Here's the drawing with two shaded views (mm, measured from the low corner). I have some questions. A direction names the side the tool comes from. Coordinates: 2 decimals unless noted, no trailing zeros. Loops run counter-clockwise (first coordinate to the right, second up) from the corner with the lowest first, then second, coordinate; pieces in that order, holes last. Notation, with made-up numbers: (70.5, -29) -> (76.5, -29) arc R26 ccw to (76.5, 8) -> close; hole circle Ø4 at (-12, 25.5). An arc over 180 degrees is marked (long way). Answer as a JSON object with one key per item and string values. Group by question number.
1) If we mould it in two halves opening along Y, with no side actions, what happens to the marked faces 3, 4 and 5? For each: +Y half, -Y half, draft (parallel to the pull), parting line (faces both ways), or undercut.
2) I'm going to push flat-ended pins straight in: pin 1 (2 mm diameter, centred on y = 11.5, z = 7.5, fed in from -X); pin 2 (5 mm diameter, centred on y = 47.5, z = 4.5, fed in from +X); pin 3 (2 mm diameter, centred on y = 7.5, z = 4.5, fed in from +X). Where does each tip first touch, or does it pass through?
3) I want a section at A-A (y = 47.5). Write out the boundary of the cut face in (x, z).
4) I want a section at C-C (x = 2.5). Write out the boundary of the cut face in (y, z), then the cut area to 3 significant figures.
5) I want a section at B-B (z = 4.25). Write out the boundary of the cut face in (x, y), then the cut area to 3 significant figures.
6) I want a section at D-D (y = 25). Write out the boundary of the cut face in (x, z).
7) Which directions (+Z, -Z, +X, -X, +Y, -Y) give clear straight access to the entire face, cutting with the end or side of a thin tool? Please do the marked faces 1 and 2.
8) I need wall thicknesses on probe 1 along Y at (x, z) = (4.2, 4.5); probe 2 along Y at (x, z) = (0.75, 4.5); probe 3 along Z at (x, y) = (3.4, 7.5). Which ranges of each line are inside material? Lowest first, please. Write a range as [from, to].
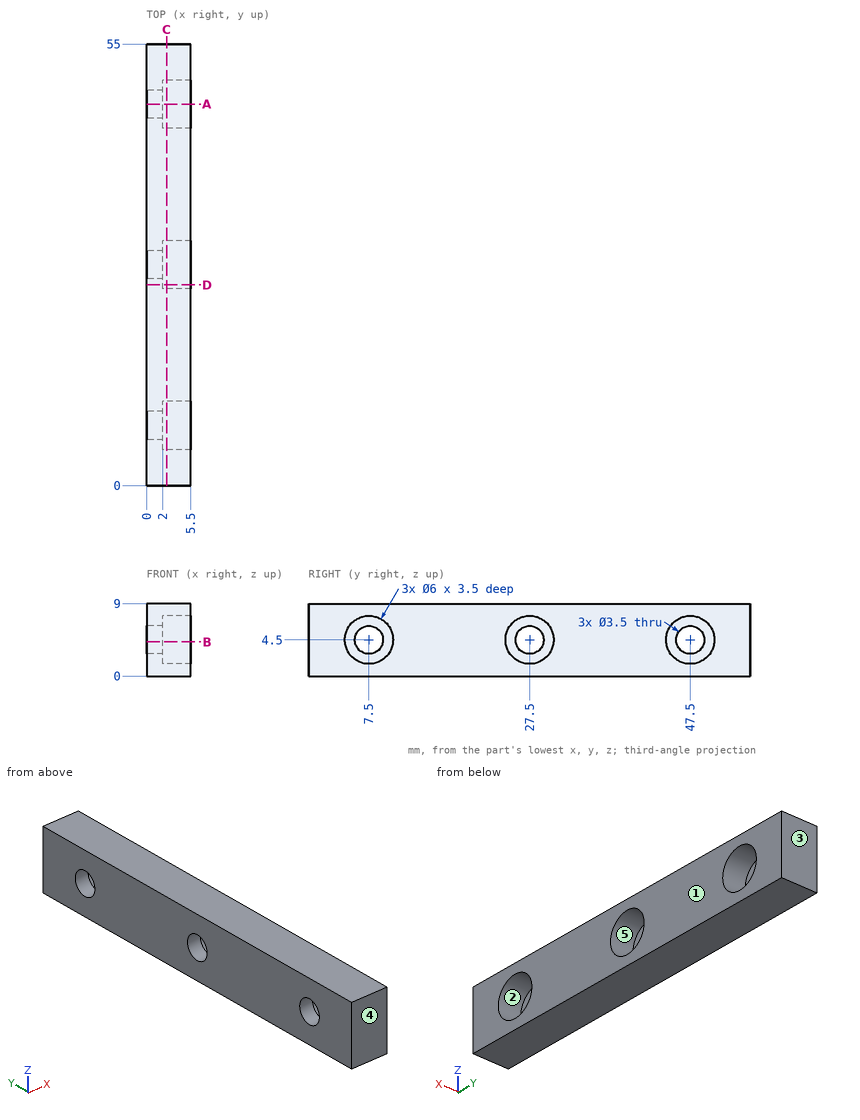
Determined:
{
 "1": {"face 3": "+Y half", "face 4": "-Y half", "face 5": "undercut"},
 "2": {"pin 1": "x = 0", "pin 2": "x = 2", "pin 3": "through"},
 "3": {"outline": "(0, 0) -> (5.5, 0) -> (5.5, 1.5) -> (2, 1.5) -> (2, 2.75) -> (0, 2.75) -> close; (0, 6.25) -> (2, 6.25) -> (2, 7.5) -> (5.5, 7.5) -> (5.5, 9) -> (0, 9) -> close"},
 "4": {"outline": "(0, 0) -> (55, 0) -> (55, 9) -> (0, 9) -> close; hole circle Ø6 at (7.5, 4.5); hole circle Ø6 at (27.5, 4.5); hole circle Ø6 at (47.5, 4.5)", "area": "410 mm^2"},
 "5": {"outline": "(0, 0) -> (5.5, 0) -> (5.5, 4.51) -> (2, 4.51) -> (2, 5.77) -> (0, 5.77) -> close; (0, 9.23) -> (2, 9.23) -> (2, 10.49) -> (5.5, 10.49) -> (5.5, 24.51) -> (2, 24.51) -> (2, 25.77) -> (0, 25.77) -> close; (0, 29.23) -> (2, 29.23) -> (2, 30.49) -> (5.5, 30.49) -> (5.5, 44.51) -> (2, 44.51) -> (2, 45.77) -> (0, 45.77) -> close; (0, 49.23) -> (2, 49.23) -> (2, 50.49) -> (5.5, 50.49) -> (5.5, 55) -> (0, 55) -> close", "area": "219 mm^2"},
 "6": {"outline": "(0, 0) -> (5.5, 0) -> (5.5, 2.84) -> (2, 2.84) -> (2, 6.16) -> (5.5, 6.16) -> (5.5, 9) -> (0, 9) -> close"},
 "7": {"face 1": "+Z, -Z, +X, +Y, -Y", "face 2": "+X"},
 "8": {"probe 1": "[0, 4.5], [10.5, 24.5], [30.5, 44.5], [50.5, 55]", "probe 2": "[0, 5.75], [9.25, 25.75], [29.25, 45.75], [49.25, 55]", "probe 3": "[0, 1.5], [7.5, 9]"}
}
